from build123d import *

# Parameters (mm, degrees)
F0_W     = 30
F0_H     = 40
F1_DEPTH = 3
F2_W     = 25
F2_H     = 35
F3_DEPTH = 3
F4_R     = 1
F5_R     = 1
F6_R     = 1.5
F7_DEPTH = 25


with BuildPart() as f1:
    # F0 (on Front) → F1 (new body)
    with BuildSketch(Plane.XZ):
        with Locations((1.927273, 10.06356)):
            Rectangle(F0_W, F0_H)
    extrude(amount=F1_DEPTH)

    # F2 (on face) → F3 (join)
    with BuildSketch(Plane.XZ.offset(3)):
        with Locations((1.927273, 10.06356)):
            Rectangle(F2_W, F2_H)
    extrude(amount=F3_DEPTH)

    # F4
    f4_edges = [f1.edges().sort_by_distance(p)[0] for p in [
        (-13.072727, -1.5, 30.06356),
        (-13.072727, -1.5, -9.93644),
        (16.927273, -1.5, -9.93644),
        (16.927273, -1.5, 30.06356),
    ]]
    fillet(f4_edges, radius=F4_R)

    # F5
    f5_edges = [f1.edges().sort_by_distance(p)[0] for p in [
        (14.427273, -6, 10.06356),
        (1.927273, -6, 27.56356),
        (-10.572727, -6, 10.06356),
        (1.927273, -6, -7.43644),
    ]]
    fillet(f5_edges, radius=F5_R)

    # F6 (on face) → F7 (cut)
    with BuildSketch(Plane.XZ.offset(6)):
        with Locations((11.427273, 17.56356)):
            Circle(F6_R)
    extrude(amount=-F7_DEPTH, mode=Mode.SUBTRACT)


solid = f1.part
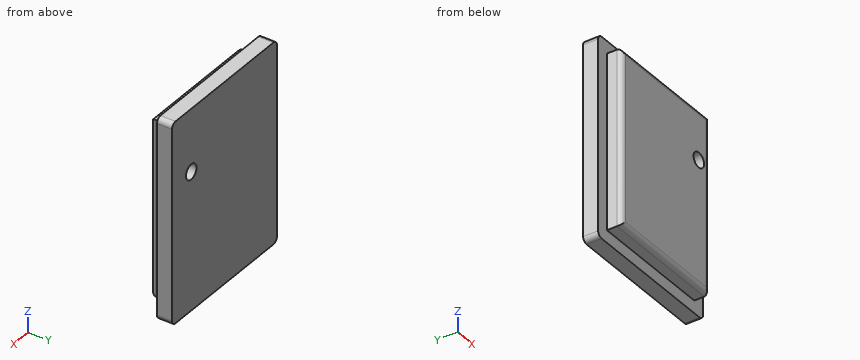
Source: CAD feature listing. Evaluate the final solid. Frame: model axes, mm. Round coordinates to 2 decimals unless told otherwise and drop trailing zeros. Loops run counter-clockwise (first coordinate to the right, second up) from the corner with the lowest first, then second, coordinate; pieces in that order, holes last.
Q1. Section C-C, the plane y = -4.3. Return loops of the section in (x, z), plus the area to 3 significant figures.
Q2. Section A-A, the plane z = 13. Return loops of the section in (x, y), plus the area to 3 significant figures.
Q3. First-contact query: P1, Ø1, axis at y = -5, z = 9, coming from the +X side; P2, Ø1.5, axis at x = 5, y = -5, coming from the -Z side; P3, Ø2, axis at y = -4.5, z = 5, coming from the -X side. Flat tips, straight axial feed; report the tip coordinate or a pass-through.
Q4. Ray query, line 1 (Z direction, x = -3, y = -5); line 2 (X direction, y = -4.6, z = 25); line 3 (Y direction, x = 15.25, z = -2). Return the intervals inside material, ascending.
Q5. Section B-B, the plane x = 6. Return loops of the section in (y, z).
Solutions:
1. outline: (-10.57, -7.44) - (14.43, -7.44) - (14.43, 27.56) - (-10.57, 27.56) - close; hole circle Ø3 at (11.43, 17.56)
1. area: 868 mm2
2. outline: (-13.07, -3) - (-10.57, -3) - (-10.57, -5) arc R1 ccw to (-9.57, -6) - (13.43, -6) arc R1 ccw to (14.43, -5) - (14.43, -3) - (16.93, -3) - (16.93, 0) - (-13.07, 0) - close
2. area: 165 mm2
3. P1: stops at x = 14.43
3. P2: stops at z = -7.44
3. P3: stops at x = -10.57
4. line 1: z = -7.44 to 27.56
4. line 2: x = -10.57 to 14.43
4. line 3: y = -3 to 0
5. outline: (-6, -6.44) arc R1 ccw to (-5, -7.44) - (-3, -7.44) - (-3, -9.94) - (0, -9.94) - (0, 30.06) - (-3, 30.06) - (-3, 27.56) - (-5, 27.56) arc R1 ccw to (-6, 26.56) - close
